Verification items for the finished model (mm, model axes). Face numbers are marked on the shaded views. A direction names the side the tool comes from. Coordinates: 2 decimals unless noted, no trailing zeros. Order: outer loops, then holes, each group sorted by start corner. A loop starts at its lowest first (then second) coordinate and runs counter-clockwise, first axis right, second up. Notation, with made-up numbers: (-14, 27) -> (39, 27) arc R26 ccw to (39, 65) -> close; hole circle Ø5 at (75, -30). An arc over 180 degrees is marked (long way). Write item = value, one per line. Start each with the question number.
1. Cross-section at D-D on z = 6.75. Record the cut outline in (x, y).
2. Cross-section at C-C on x = 90. Record the cut outline in (y, z).
3. Thickness scan on line 1 along X through (y, z) = (-68, 10.5); line 2 along Y through (x, z) = (30.5, 8.25); line 3 along X through (y, z) = (-20.5, 3). Record the ranges inside material, lowest first. Write a range as from..to.
4. Release check for a two-part mould opening along Y. For the marked faces 4, 5 and 6 record: +Y half, -Y half, draft (parallel to the pull), parting line (faces both ways), or undercut.
5. Set-up check for the marked faces 1, 2 and 3: record each of +Z, -Z, +X, -X, +Y, -Y from which the full face is reachable in a straight line by a thin tool's end or side.
6. Cross-section at B-B on x = 13. Record the cut outline in (y, z), plus the area to 3 significant figures.
7. Cross-section at A-A on y = -20.5. Record the cut outline in (x, z), plus the area to 3 significant figures.
8. Go/stop test with flat-tipped pins: P1, Ø4.5, axis at y = -66, z = 7, coming from the -X side; P2, Ø2, axis at x = 66.5, z = 19, coming from the +Y side; P3, Ø8, axis at x = 84.5, z = 18.5, coming from the -Y side; P4, Ø5, axis at x = 46.5, y = -47, coming from the +Z side. Record where each tip stops, or that it passes through.
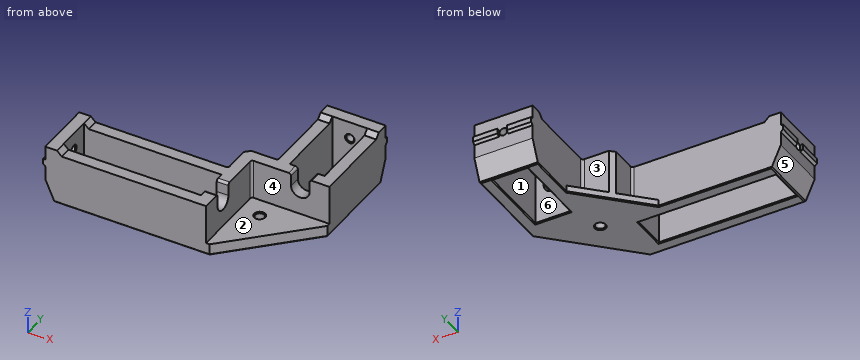
from build123d import *

# Parameters (mm, degrees)
SKETCH005_R        = 2
SKETCH005_W        = 59
SKETCH005_H        = 15
SKETCH005_W_2      = 15
SKETCH005_H_2      = 31.5
PAD002_DEPTH       = 24
SKETCH007_W        = 33.5
SKETCH007_H        = 33.5
POCKET003_DEPTH    = 19
CHAMFER002004_SIZE = 32
SKETCH008_W        = 95.5
SKETCH008_H        = 68
POCKET004_DEPTH    = 2
CHAMFER002005_SIZE = 1.99
POCKET005_DEPTH    = 75.001
POCKET006_DEPTH    = 102.501
POCKET007_DEPTH    = 19
SKETCH012_R        = 1.65
POCKET008_DEPTH    = 5
SKETCH013_R        = 1.65
POCKET009_DEPTH    = 5
SKETCH014_W        = 10.5
SKETCH014_H        = 3.2
PAD003_DEPTH       = 1
SKETCH015_W        = 10.5
SKETCH015_H        = 3.2
PAD004_DEPTH       = 1
CHAMFER002006_SIZE = 0.99
POCKET010_DEPTH    = 5
POCKET011_DEPTH    = 5
CHAMFER002007_SIZE = 0.4
FILLET001002_R     = 1
CHAMFER002008_SIZE = 0.4


with BuildPart() as part:
    # Sketch005 → Pad002 (new body)
    with BuildSketch(Plane.XY):
        Polygon((52.5, -50), (77.5, -25), (77.5, 0), (102.5, 0), (102.5, -75), (0, -75), (0, -50), align=None)
        with Locations((77.5, -50)):
            Circle(SKETCH005_R, mode=Mode.SUBTRACT)
        with Locations((34.5, -62.5)):
            Rectangle(SKETCH005_W, SKETCH005_H, mode=Mode.SUBTRACT)
        with Locations((90, -20.75)):
            Rectangle(SKETCH005_W_2, SKETCH005_H_2, mode=Mode.SUBTRACT)
    extrude(amount=PAD002_DEPTH)

    # Sketch007 (on Face18 of Pad002) → Pocket003 (cut)
    with BuildSketch(Plane.XY.offset(24)):
        with Locations((85.75, -58.25)):
            Rectangle(SKETCH007_W, SKETCH007_H)
    extrude(amount=-POCKET003_DEPTH, mode=Mode.SUBTRACT)

    # Chamfer002004
    chamfer002004_edges = [part.edges().sort_by_distance(p)[0] for p in [
        (102.5, -75, 2.5),
    ]]
    chamfer(chamfer002004_edges, length=CHAMFER002004_SIZE)

    # Sketch008 (on Face6 of Chamfer002004) → Pocket004 (cut)
    with BuildSketch(Plane.XY.offset(24)):
        with Locations((54.75, -41)):
            Rectangle(SKETCH008_W, SKETCH008_H)
    extrude(amount=-POCKET004_DEPTH, mode=Mode.SUBTRACT)

    # Chamfer002005
    chamfer002005_edges = [part.edges().sort_by_distance(p)[0] for p in [
        (7, -72.5, 24),
        (7, -52.5, 24),
        (80, -7, 24),
        (100, -7, 24),
    ]]
    chamfer(chamfer002005_edges, length=CHAMFER002005_SIZE)

    # Sketch009 (on Face1 of Chamfer002005) → Pocket005 (cut, through all)
    with BuildSketch(Plane.XZ.offset(75)):
        Polygon((0, 9), (4, 0), (0, 0), align=None)
    extrude(amount=-POCKET005_DEPTH, mode=Mode.SUBTRACT)

    # Sketch010 (on Face17 of Pocket005) → Pocket006 (cut, through all)
    with BuildSketch(Plane.YZ.offset(102.5)):
        Polygon((0, 9), (-4, 0), (0, 0), align=None)
    extrude(amount=-POCKET006_DEPTH, mode=Mode.SUBTRACT)

    # Sketch011 (on Face10 of Pocket006) → Pocket007 (cut)
    with BuildSketch(Plane.XY.offset(22)):
        Polygon((64, -38.5), (64, -50), (52.5, -50), align=None)
        Polygon((77.5, -25), (77.5, -36.5), (66, -36.5), align=None)
    extrude(amount=-POCKET007_DEPTH, mode=Mode.SUBTRACT)

    # Sketch012 (on Face4 of Pocket007) → Pocket008 (cut)
    with BuildSketch(Plane(origin=(0, 0, 0), x_dir=(0, -1, 0), z_dir=(-1, 0, 0))):
        with Locations((62.5, 16.5)):
            Circle(SKETCH012_R)
    extrude(amount=-POCKET008_DEPTH, mode=Mode.SUBTRACT)

    # Sketch013 (on Face37 of Pocket008) → Pocket009 (cut)
    with BuildSketch(Plane(origin=(0, 0, 0), x_dir=(-1, 0, 0), z_dir=(0, 1, 0))):
        with Locations((-90, 16.5)):
            Circle(SKETCH013_R)
    extrude(amount=-POCKET009_DEPTH, mode=Mode.SUBTRACT)

    # Sketch014 (on Face37 of Pocket009) → Pad003 (join)
    with BuildSketch(Plane(origin=(0, 0, 0), x_dir=(-1, 0, 0), z_dir=(0, 1, 0))):
        with Locations((-97.25, 16.5)):
            Rectangle(SKETCH014_W, SKETCH014_H)
        with Locations((-82.75, 16.5)):
            Rectangle(SKETCH014_W, SKETCH014_H)
    extrude(amount=PAD003_DEPTH)

    # Sketch015 (on Face4 of Pad003) → Pad004 (join)
    with BuildSketch(Plane(origin=(0, 0, 0), x_dir=(0, -1, 0), z_dir=(-1, 0, 0))):
        with Locations((55.25, 16.5)):
            Rectangle(SKETCH015_W, SKETCH015_H)
        with Locations((69.75, 16.5)):
            Rectangle(SKETCH015_W, SKETCH015_H)
    extrude(amount=PAD004_DEPTH)

    # Chamfer002006
    chamfer002006_edges = [part.edges().sort_by_distance(p)[0] for p in [
        (-1, -55.25, 14.9),
        (-1, -69.75, 14.9),
        (97.25, 1, 14.9),
        (82.75, 1, 14.9),
    ]]
    chamfer(chamfer002006_edges, length=CHAMFER002006_SIZE)

    # Sketch016 (on Face15 of Chamfer002006) → Pocket010 (cut)
    with BuildSketch(Plane.YZ.offset(69)):
        with BuildLine():
            ThreePointArc((-66.5, 16.5), (-62.5, 12.5), (-58.5, 16.5))
            Line((-58.5, 24), (-58.5, 16.5))
            Line((-66.5, 24), (-58.5, 24))
            Line((-66.5, 16.5), (-66.5, 24))
        make_face()
    extrude(amount=-POCKET010_DEPTH, mode=Mode.SUBTRACT)

    # Sketch017 (on Face37 of Pocket010) → Pocket011 (cut)
    with BuildSketch(Plane.XZ.offset(41.5)):
        with BuildLine():
            ThreePointArc((86, 16.5), (90, 12.5), (94, 16.5))
            Line((94, 24), (94, 16.5))
            Line((86, 24), (94, 24))
            Line((86, 16.5), (86, 24))
        make_face()
    extrude(amount=-POCKET011_DEPTH, mode=Mode.SUBTRACT)

    # Chamfer002007
    chamfer002007_edges = [part.edges().sort_by_distance(p)[0] for p in [
        (102.5, -23.5, 0),
        (90, -4, 0),
        (77.5, -14.5, 0),
        (65, -37.5, 0),
        (28.25, -50, 0),
        (4, -62.5, 0),
        (37.25, -75, 0),
        (86.5, -59, 0),
        (75.5, -50, 0),
        (5, -62.5, 0),
        (34.5, -70, 0),
        (34.5, -55, 0),
        (64, -62.5, 0),
        (82.5, -20.75, 0),
        (90, -36.5, 0),
        (90, -5, 0),
        (97.5, -20.75, 0),
        (75.5, -50, 5),
    ]]
    chamfer(chamfer002007_edges, length=CHAMFER002007_SIZE)

    # Fillet001002
    fillet001002_edges = [part.edges().sort_by_distance(p)[0] for p in [
        (66.5, -66.5, 22),
        (66.5, -58.5, 22),
        (86, -39, 22),
        (94, -39, 22),
        (69, -41.5, 13.5),
        (64, -50, 12.5),
        (77.5, -36.5, 12.5),
    ]]
    fillet(fillet001002_edges, radius=FILLET001002_R)

    # Chamfer002008
    chamfer002008_edges = [part.edges().sort_by_distance(p)[0] for p in [
        (5, -60.85, 16.5),
        (91.65, -5, 16.5),
    ]]
    chamfer(chamfer002008_edges, length=CHAMFER002008_SIZE)


solid = part.part
Worked out:
q1.outline = (1, -75) -> (69, -75) -> (69, -42.5) arc R1 cw to (70, -41.5) -> (102.5, -41.5) -> (102.5, -1) -> (77.5, -1) -> (77.5, -35.5) arc R1 cw to (76.5, -36.5) -> (66, -36.5) -> (64, -38.5) -> (64, -49) arc R1 cw to (63, -50) -> (1, -50) -> close; hole (5, -70) -> (64, -70) -> (64, -55) -> (5, -55) -> close; hole (82.5, -36.5) -> (97.5, -36.5) -> (97.5, -5) -> (82.5, -5) -> close
q2.outline = (-55.5, 0.4) -> (-54.93, 0) -> (-36.9, 0) -> (-36.5, 0.4) -> (-36.5, 12.5) -> (-41.5, 12.5) -> (-41.5, 5) -> (-55.5, 5) -> close; (-5, 0.4) -> (-4.6, 0) -> (-4.4, 0) -> (-3.84, 0.37) -> (0, 9) -> (0, 14.85) -> (-4.6, 14.85) -> (-5, 14.45) -> close; (-5, 18.55) -> (-4.6, 18.15) -> (0, 18.15) -> (0, 24) -> (-5, 24) -> close
q3.line_1 = 0..5, 64..69
q3.line_2 = -75..-70, -55..-50
q3.line_3 = 77.5..82.5, 97.5..102.5
q4.face_4 = -Y half
q4.face_5 = draft
q4.face_6 = undercut
q5.face_1 = +Z, -Z
q5.face_2 = +Z, +X, -Y
q5.face_3 = +Z, -X, +Y
q6.outline = (-75, 0.4) -> (-74.6, 0) -> (-70.4, 0) -> (-70, 0.4) -> (-70, 22) -> (-75, 22) -> close; (-55, 0.4) -> (-54.6, 0) -> (-50.4, 0) -> (-50, 0.4) -> (-50, 22) -> (-55, 22) -> close
q6.area = 220 mm²
q7.outline = (77.5, 0.4) -> (77.9, 0) -> (82.1, 0) -> (82.5, 0.4) -> (82.5, 22) -> (77.5, 22) -> close; (97.5, 0.4) -> (97.9, 0) -> (102.1, 0) -> (102.5, 0.4) -> (102.5, 22) -> (97.5, 22) -> close
q7.area = 220 mm²
q8.P1 = 0
q8.P2 = -36.5
q8.P3 = -41.5
q8.P4 = through
